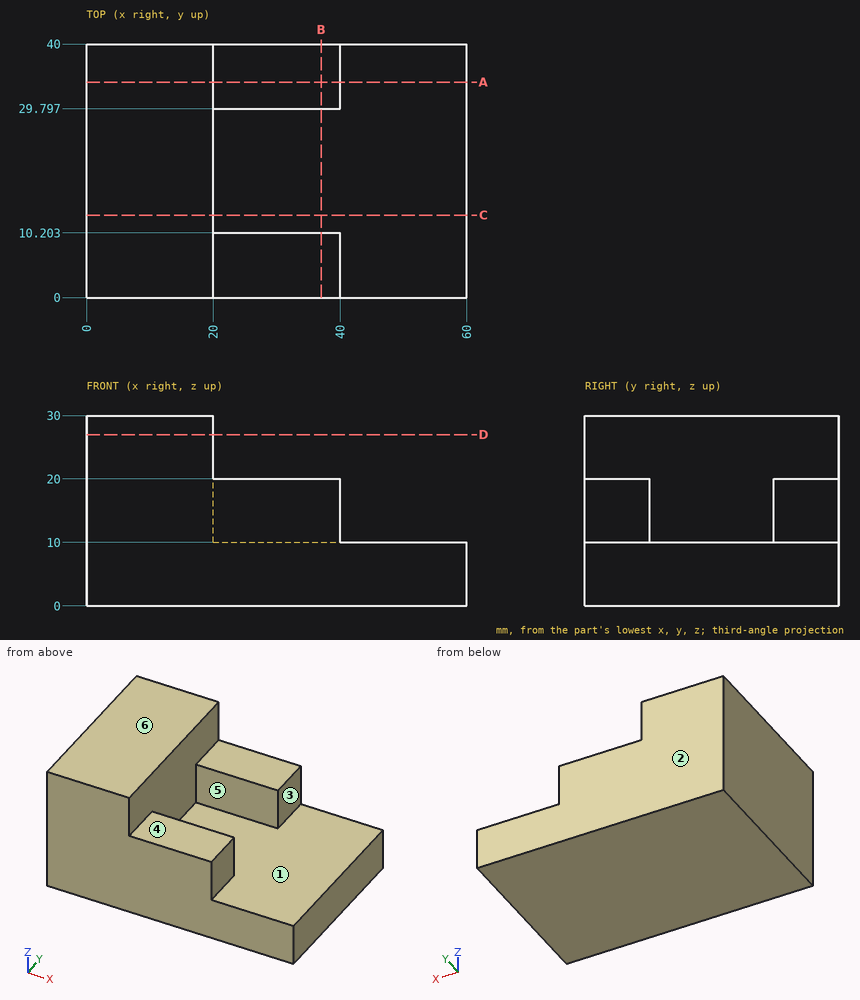
Answer from the drawing. Dimensions are ordinates in mm from the lowest x, y and z of the part. A direction names the side the tool comes from. Give positions to 0.01 mm unless a question says otherwise; leave off trailing zeros. Write each loop counter-clockwise with the first axis right and the second up, starting at its lowest first coordinate (ties: lowest second). Pieces come first, ordered by that corner, then holes. Notation, with made-up numbers: (82.5, 83.5) -> (133.5, 83.5) arc R28 ccw to (133.5, 117.5) -> close; hole circle Ø7 at (35, 79.25). An arc over 180 degrees is marked (long way). Use a Markdown table: item, result.
(1) Section D-D, the plane z = 27 is taken. Determine the outline of the cut face in (x, y).
Return value:
| item | result |
|---|---|
| outline | (0, 0) -> (20, 0) -> (20, 40) -> (0, 40) -> close |
(2) Flat-ended cylindrical pins translate along their axes: P1, Ø12, axis at x = 34, y = 18, coming from the +Z side; P2, Ø3, axis at x = 29, y = 3, coming from the +Z side; P3, Ø16, axis at y = 29.5, z = 23, coming from the +X side. Find the tip coordinate at first contact, or state that the pin passes through.
Return value:
| item | result |
|---|---|
| P1 | z = 10 |
| P2 | z = 20 |
| P3 | x = 40 |
(3) Section C-C, the plane y = 13 is taken. Determine the outline of the cut face in (x, z), then the cut area to 3 significant figures.
Return value:
| item | result |
|---|---|
| outline | (0, 0) -> (60, 0) -> (60, 10) -> (20, 10) -> (20, 30) -> (0, 30) -> close |
| area | 1,000 mm2 |
(4) Section A-A, the plane y = 34 is taken. Determine the outline of the cut face in (x, z).
Return value:
| item | result |
|---|---|
| outline | (0, 0) -> (60, 0) -> (60, 10) -> (40, 10) -> (40, 20) -> (20, 20) -> (20, 30) -> (0, 30) -> close |
(5) For the marked faces 4, 5 and 6, determine the directions among +Z, -Z, +X, -X, +Y, -Y from which every point of the face is accessible in a straight line to the end or side of a thin tool.
Return value:
| item | result |
|---|---|
| face 4 | +Z, +X, +Y, -Y |
| face 5 | +Z, +X |
| face 6 | +Z, +X, -X, +Y, -Y |
(6) Find the intervals of material crossed by probe 1 along Y at (x, z) = (36, 17.5); probe 2 along X at (y, z) = (18.5, 28.5); probe 3 along Z at (x, y) = (46.5, 24), in increasing order. Write a range as from..to.
Return value:
| item | result |
|---|---|
| probe 1 | 0..10.2, 29.8..40 |
| probe 2 | 0..20 |
| probe 3 | 0..10 |
(7) Section B-B, the plane x = 37 is taken. Determine the outline of the cut face in (y, z), then the cut area to 3 significant figures.
Return value:
| item | result |
|---|---|
| outline | (0, 0) -> (40, 0) -> (40, 20) -> (29.8, 20) -> (29.8, 10) -> (10.2, 10) -> (10.2, 20) -> (0, 20) -> close |
| area | 604 mm2 |
(8) Determine the mould class of the marked faces 1, 2 and 3 for opening direction Y: released by +Y, released by -Y, zero draft, split by the parting line, or undercut.
Return value:
| item | result |
|---|---|
| face 1 | undercut |
| face 2 | released by +Y |
| face 3 | zero draft |
